Here's the drawing with two shaded views (mm, measured from the low corner). I have some questions. Give positions to 0.01 mm unless a question says otherwise; leave off trailing zeros. Write each loop counter-clockwise with the first axis right and the second up, starting at its lowest first coordinate (ties: lowest second). Pieces come first, ordered by that corner, then holes. Notation, with made-up numbers: (9, 46.25) -> (54, 46.25) arc R22 ccw to (54, 66.25) -> close; hole circle Ø9 at (70.5, -27). An arc over 180 degrees is marked (long way). One line per question, with ' | ' between items.
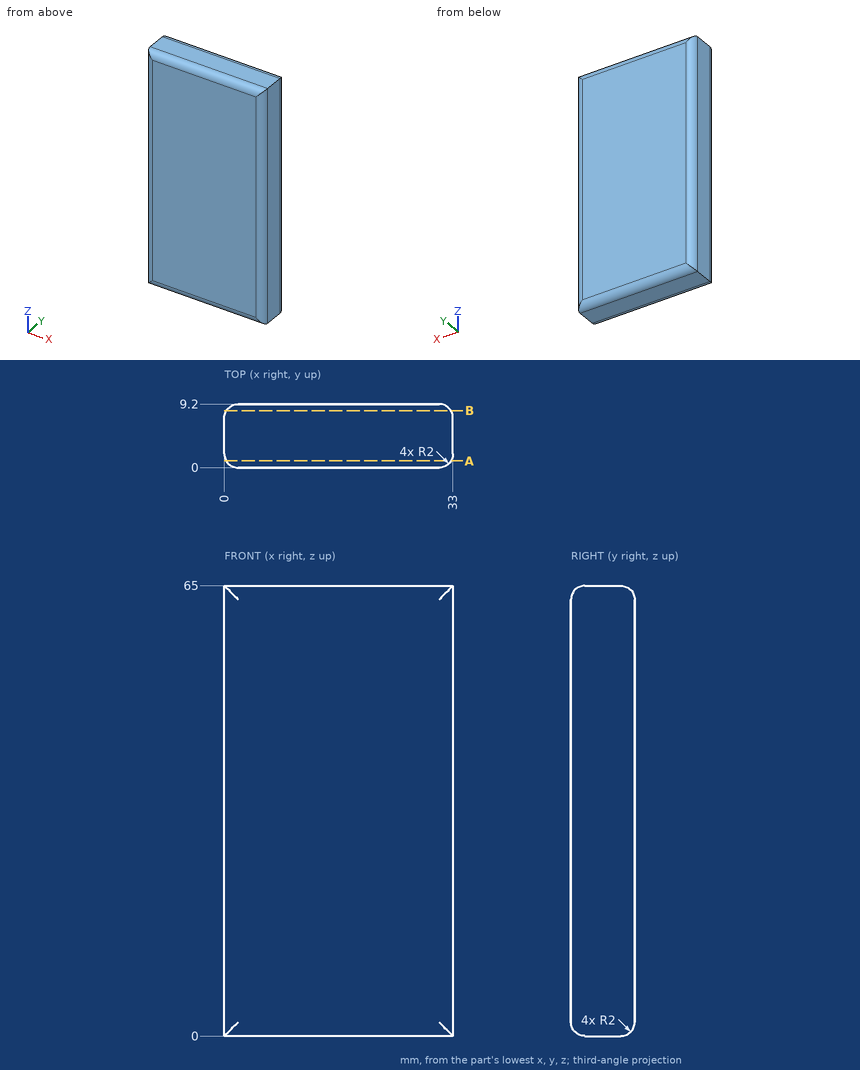
Q1. If I drill on line 1 along Z through (x, y) = (18, 1.25); line 2 along X through (y, z) = (9, 8.5); line 3 along Z through (x, y) = (31.5, 1), over which ranges is the centre line in solid material (lowest first)?
Answer below:
line 1: z = 0.15 to 64.85 | line 2: x = 1.13 to 31.87 | line 3: z = 0.27 to 64.73
Q2. Imagine slicing it at B-B on y = 8.25. Please give me the cut outline in (x, z).
Answer below:
outline: (0.3, 0.3) -> (32.7, 0.3) -> (32.7, 64.7) -> (0.3, 64.7) -> close
Q3. Imagine slicing it at A-A on y = 1. Please give me the cut outline in (x, z), and give its area (3 significant figures).
Answer below:
outline: (0.27, 0.27) -> (32.73, 0.27) -> (32.73, 64.73) -> (0.27, 64.73) -> close | area: 2,090 mm^2
